The model under review builds one solid part; all positions refer to its coordinate system, in mm. Coordinates: 2 decimals unless noted, no trailing zeros. Order: outer loops, then holes, each group sorted by start corner. A loop starts at its lowest first (then second) coordinate and runs counter-clockwise, first axis right, second up. Notation, with made-up numbers: M 29.5,-18.75 L 53.5,-18.75 A12 ccw 53.5,2.25 Z; hole C 54.25,89.5 d11. An arc over 180 degrees is marked long. Answer as CSV lines item,"result". Start each with the question number.
Q1. Wall thickness on L1, parallel to X at y = -3.25, z = -17; L2, parallel to Z at x = 14, y = -2; L3, parallel to Z at x = 29.5, y = -2.25: over which ranges is each line inside the solid? List them lowest first. Write a range as [from, to].
Q2. Consider section B-B on x = 36. Write out the cut boundary in (y, z).
Q3. Consider section A-A on y = -2.6. Write out the cut boundary in (x, z).
Q4. For P1, Ø2, axis at x = 24, y = -2.5, coming from the -Z side, flat-tipped, find the tip position at first contact; note if it passes through.
Q5. Consider section C-C on z = -15.5. Write out the cut boundary in (x, y).
from build123d import *

# Parameters (mm, degrees)
F1_DEPTH = 4


with BuildPart() as f1:
    # F0 (on Front) → F1 (new body)
    with BuildSketch(Plane.XZ):
        with BuildLine():
            Line((60, 0), (9.287088, 0))
            ThreePointArc((9.287088, 0), (8.030526, -0.444027), (7.331911, -1.578947))
            ThreePointArc((7.331911, -1.578947), (5.303301, -5.303301), (1.578947, -7.331911))
            ThreePointArc((1.578947, -7.331911), (0.444027, -8.030526), (0, -9.287088))
            Line((0, -9.287088), (0, -60))
            ThreePointArc((0, -60), (42.426407, -42.426407), (60, 0))
        make_face()
    extrude(amount=F1_DEPTH)


solid = f1.part
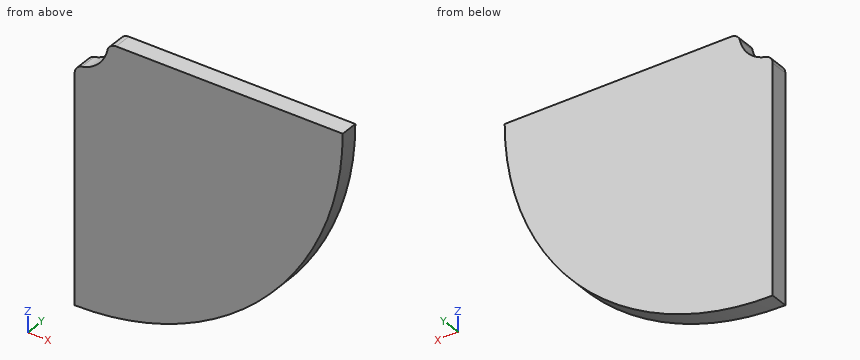
Evaluation:
1,L1,"x = [0, 57.54]"
1,L2,"z = [-58.34, 0]"
1,L3,"z = [-52.25, 0]"
2,outline,"M -4,-48 L 0,-48 L 0,0 L -4,0 Z"
3,outline,"M 0,-60 A60 ccw 60,0 L 9.29,0 A2 ccw 7.33,-1.58 A7.5 cw 1.58,-7.33 A2 ccw 0,-9.29 Z"
4,P1,"stops at z = -55.42"
5,outline,"M 0,-4 L 57.96,-4 L 57.96,0 L 0,0 Z"
